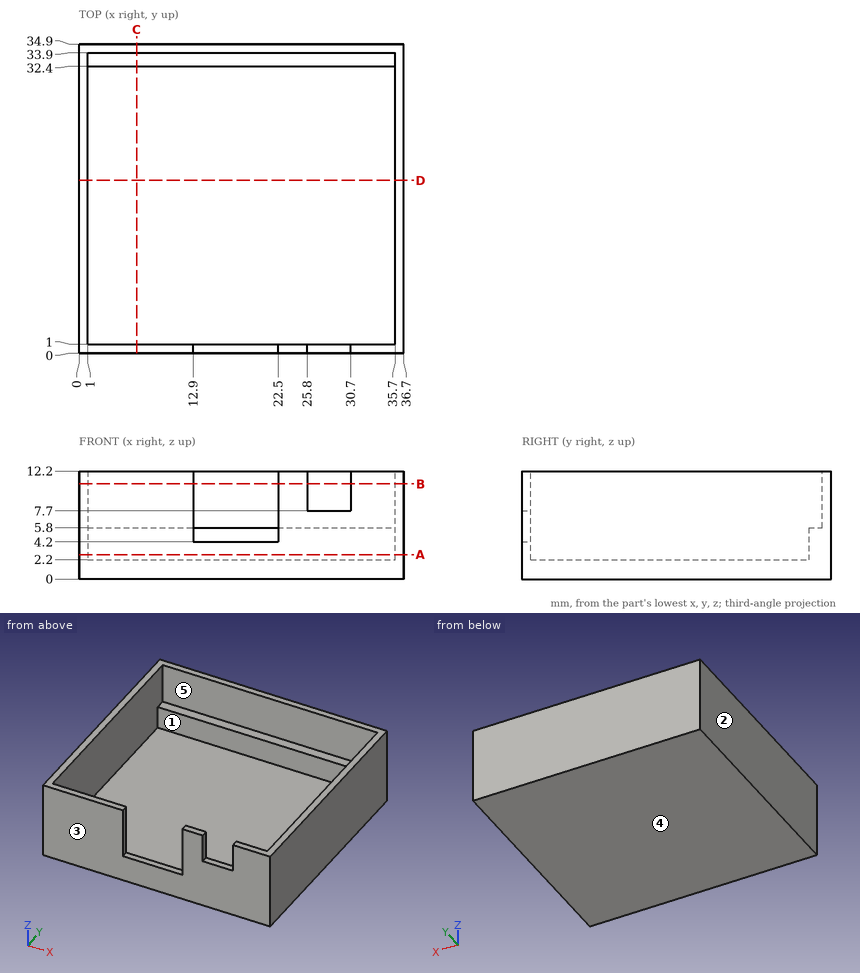
Could you check a few things on this drawing? It's one solid part, dimensions in mm from its lowest x, y, z. A direction names the side the tool comes from. Coordinates: 2 decimals unless noted, no trailing zeros. Order: outer loops, then holes, each group sorted by start corner. A loop starts at its lowest first (then second) coordinate and runs counter-clockwise, first axis right, second up. Notation, with made-up numbers: (-21.75, 34.25) - (9.25, 34.25) arc R31 cw to (9.25, 66.25) - close; hole circle Ø10 at (51.5, 56). An arc over 180 degrees is marked (long way). One line per question, with ' | ' between items. Start each with the question number.
1. If we section it at B-B (z = 10.75): Write out the boundary of the cut face in (x, y), and give its area (3 significant figures).
2. If we section it at A-A (z = 2.75): Write out the boundary of the cut face in (x, y).
3. If we mould it in two halves opening along X, with no side actions, what happens to the marked faces 1, 2 and 3? For each: released by +X, released by -X, zero draft, split by the parting line, or undercut.
4. If we section it at C-C (x = 6.5): Write out the boundary of the cut face in (y, z).
5. If we section it at D-D (y = 19.5): Write out the boundary of the cut face in (x, z).
6. I'm going to push flat-ended pins straight in: pin 1 Ø3 at (x, z) = (15, 9.5) entering from -Y; pin 2 Ø5 at (x, y) = (12.5, 30.5) entering from +Z; pin 3 Ø0.5 at (x, y) = (19, 0.5) entering from +Z. Where does each tip first touch, or does it pass through?
7. Which directions (+Z, -Z, +X, -X, +Y, -Y) give clear straight access to the entire face, cutting with the end or side of a thin tool? Please do the marked faces 4 and 5.
8. Please list where these lines run through material, in increasing order: line 1 along X through (y, z) = (21.5, 4.5); line 2 along Y through (x, z) = (10, 8.5); line 3 along Y through (x, z) = (26, 4.75). Write a range as [from, to].
Model answer:
1) outline: (0, 0) - (12.9, 0) - (12.9, 1) - (1, 1) - (1, 33.9) - (35.7, 33.9) - (35.7, 1) - (30.7, 1) - (30.7, 0) - (36.7, 0) - (36.7, 34.9) - (0, 34.9) - close; (22.5, 0) - (25.8, 0) - (25.8, 1) - (22.5, 1) - close | area: 125 mm²
2) outline: (0, 0) - (36.7, 0) - (36.7, 34.9) - (0, 34.9) - close; hole (1, 1) - (35.7, 1) - (35.7, 32.4) - (1, 32.4) - close
3) face 1: undercut | face 2: released by -X | face 3: zero draft
4) outline: (0, 0) - (34.9, 0) - (34.9, 12.2) - (33.9, 12.2) - (33.9, 5.8) - (32.4, 5.8) - (32.4, 2.2) - (1, 2.2) - (1, 12.2) - (0, 12.2) - close
5) outline: (0, 0) - (36.7, 0) - (36.7, 12.2) - (35.7, 12.2) - (35.7, 2.2) - (1, 2.2) - (1, 12.2) - (0, 12.2) - close
6) pin 1: stops at y = 33.9 | pin 2: stops at z = 5.8 | pin 3: stops at z = 4.2
7) face 4: -Z, +X, -X, +Y, -Y | face 5: +Z
8) line 1: x = [0, 1], [35.7, 36.7] | line 2: y = [0, 1], [33.9, 34.9] | line 3: y = [0, 1], [32.4, 34.9]
